Input: dimensioned drawing with shaded views. Units: mm. Origin: part minimum x, y, z. A direction names the side the tool comes from. Round coordinates to 2 decimals unless told otherwise and drop trailing zeros. Loops run counter-clockwise (first coordinate to the right, second up) from the corner with the lowest first, then second, coordinate; pieces in that order, holes last. Notation, with made-up numbers: (-33, -17.5) - (12, -17.5) arc R24 cw to (12, -2.5) - close; hole circle Ø5 at (54, 80.25). An arc over 180 degrees is marked (long way). Write each question's results on one line, items separated by ' | '.
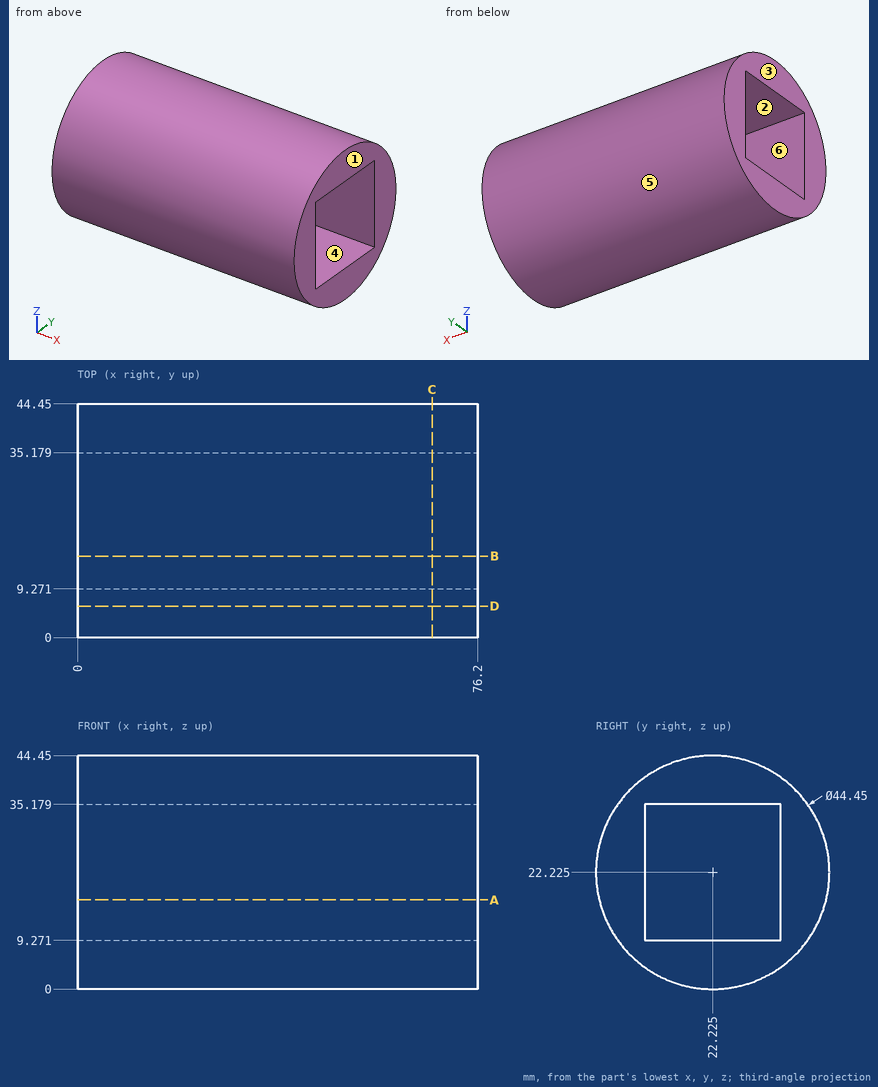
1. Line query: line 1 (Z direction, x = 50.5, y = 21.5); line 2 (Y direction, x = 30, z = 15.5); line 3 (Z direction, x = 11, y = 27.5). Output: solid intervals per line, ascending. Write a range as [from, to].
Answer:
line 1: [0.01, 9.27], [35.18, 44.44] | line 2: [1.04, 9.27], [35.18, 43.41] | line 3: [0.64, 9.27], [35.18, 43.81]
2. Set-up query: the marked faces 1 and 2. Return all of +Z, -Z, +X, -X, +Y, -Y with unobstructed straight access to the full face (end or side cutting, diameter ignored); none if empty.
Answer:
face 1: +Z, -Z, +X, +Y, -Y | face 2: +X, -X
3. Mould query, pull axis Z, two halves, no side actions, for the marked faces 3, 4, 5 and 6. Classes: pulls with the +Z half, pulls with the -Z half, needs draft (parallel to the pull), parting line crosses it, or undercut.
Answer:
face 3: needs draft | face 4: undercut | face 5: parting line crosses it | face 6: undercut
4. Section query B-B, the plane y = 15.5. Output: boundary loops of the cut face in (x, z), plus the area to 3 significant figures.
Answer:
outline: (0, 1.04) - (76.2, 1.04) - (76.2, 9.27) - (0, 9.27) - close; (0, 35.18) - (76.2, 35.18) - (76.2, 43.41) - (0, 43.41) - close | area: 1,250 mm^2
5. Section query A-A, the plane z = 17. Output: boundary loops of the cut face in (x, y).
Answer:
outline: (0, 0.62) - (76.2, 0.62) - (76.2, 9.27) - (0, 9.27) - close; (0, 35.18) - (76.2, 35.18) - (76.2, 43.83) - (0, 43.83) - close
6. Contact query for flat-ended pins moving along their axis: pin 1 (8 mm diameter, centred on x = 31.5, y = 24, fed in from -Z); pin 2 (1.5 mm diameter, centred on x = 55.5, z = 10.5, fed in from -Y); pin 3 (6 mm diameter, centred on x = 27.5, y = 18.5, fed in from +Z). Output: stop coordinate, or through.
Answer:
pin 1: z = 0 | pin 2: y = 2.9 | pin 3: z = 44.44
7. Section query D-D, the plane y = 6. Output: boundary loops of the cut face in (x, z).
Answer:
outline: (0, 7.04) - (76.2, 7.04) - (76.2, 37.41) - (0, 37.41) - close
8. Section query C-C, the plane x = 67.5. Output: boundary loops of the cut face in (y, z) (3 decimals).
Answer:
outline: circle Ø44.45 at (22.225, 22.225); hole (9.271, 9.271) - (35.179, 9.271) - (35.179, 35.179) - (9.271, 35.179) - close
